Geometry: see drawing. Coordinates: mm, zero at the bounding-box minimum. A direction names the side the tool comes from. Round coordinates to 2 decimals unless told otherwise and drop trailing zeros. Write each loop counter-clockwise with the first axis right and the second up, starting at its lowest first coordinate (ties: lowest second). Pieces come first, ordered by that corner, then holes. Notation, with made-up numbers: M 83.25,26 L 132.25,26 A14 ccw 132.25,34 Z; hole C 31,54 d5. An arc over 180 degrees is marked long. Use one line per item in the form item = value. Start each with the question number.
Item 1: Ray query, probe 1 along Z at (x, y) = (11.25, 4.25); probe 2 along X at (y, z) = (7.25, 16.75); probe 3 along Y at (x, z) = (10.5, 1.75). Return the intervals inside material, ascending.
Item 2: Section query A-A (x = 21.75). Return loops of the section in (y, z).
Item 3: Section query B-B (y = 8.75). Return loops of the section in (x, z), and give its area (3 significant figures).
Item 4: Section query D-D (x = 18). Return loops of the section in (y, z).
Item 5: Section query C-C (z = 11.5). Return loops of the section in (x, y).
Item 6: Reachability of the marked faces 1, 2 and 3 from +Z, -Z, +X, -X, +Y, -Y: full face, straight path, thin tool, end or side. Return the list, or none.
Item 7: Pin query (flat end, axial travel): pin 1 Ø11 at (x, z) = (8, 7) entering from +Y; pin 2 Ø11 at (y, z) = (16.5, 15.5) entering from -X. Return the tip coordinate at first contact, or that it passes through.
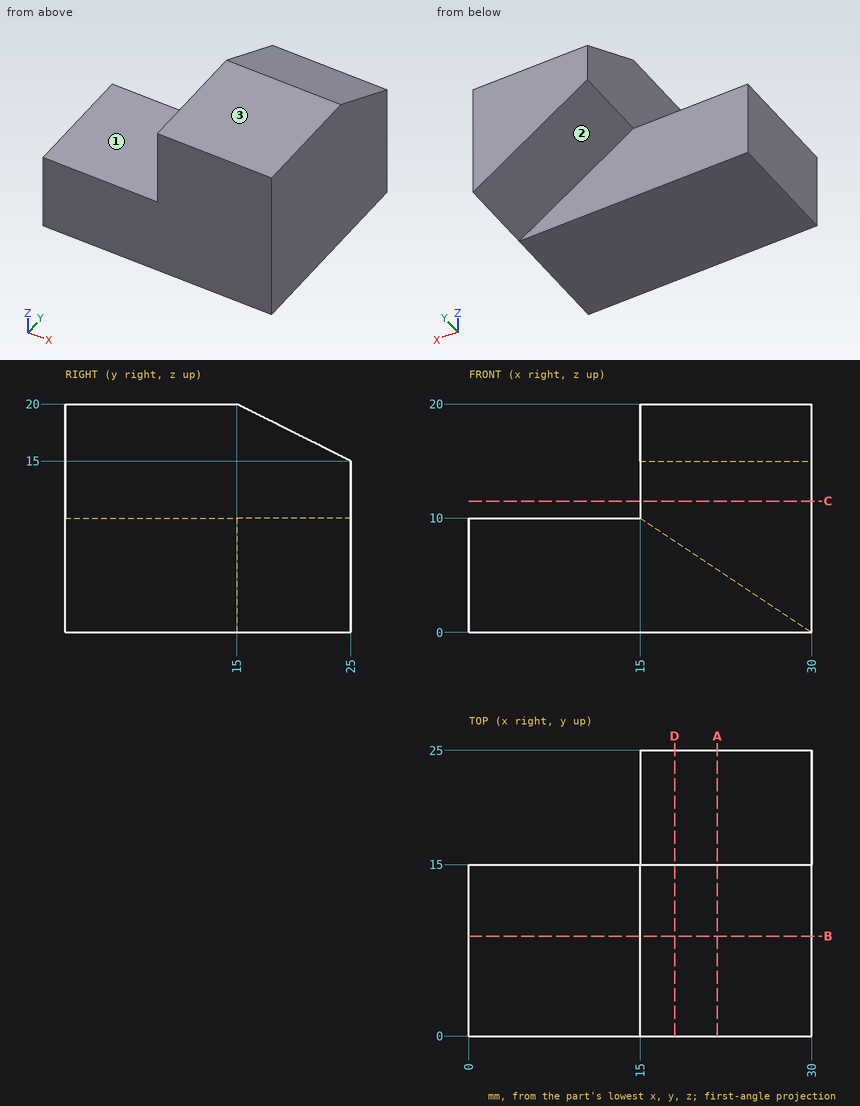
Working result:
q1.probe_1 = 0 to 10
q1.probe_2 = 15 to 30
q1.probe_3 = 0 to 15
q2.outline = M 0,0 L 15,0 L 15,5.5 L 25,5.5 L 25,15 L 15,20 L 0,20 Z
q3.outline = M 0,0 L 30,0 L 30,20 L 15,20 L 15,10 L 0,10 Z
q3.area = 450 mm²
q4.outline = M 0,0 L 15,0 L 15,8 L 25,8 L 25,15 L 15,20 L 0,20 Z
q5.outline = M 15,0 L 30,0 L 30,25 L 15,25 Z
q6.face_1 = +Z, -X, +Y, -Y
q6.face_2 = -Z, -X, +Y
q6.face_3 = +Z, +X, -X, +Y, -Y
q7.pin_1 = 15
q7.pin_2 = 15
